```python
from build123d import *

# Parameters (mm, degrees)
F0_R         = 28.5
F0_R_2       = 18.5
F1_DEPTH     = 15
F2_R         = 28.5
F2_R_2       = 18.5
F3_DEPTH     = 5
F4_R         = 2
F4_R_2       = 11.2
F5_DEPTH     = 25
F7_DEPTH     = 65
F8_W         = 40
F8_H         = 5
F9_DEPTH     = 18
F10_R        = 3.2
F11_DEPTH    = 25
F12_W        = 18
F12_H        = 3
F13_DEPTH    = 60
F14_C1_SIZE2 = 60
F14_C1_SIZE  = 18
F14_C2_SIZE2 = 60
F14_C2_SIZE  = 18
F14_C3_SIZE2 = 60
F14_C3_SIZE  = 18
F14_C4_SIZE2 = 60
F14_C4_SIZE  = 18


# Not quite as in the source:
# - a pattern or mirror of a feature is missing from the dataset's text; its kind, count and spacing are read off the source's solid
# - a feature names something its author has since deleted; it is built from what else it names


with BuildPart() as f1:
    # F0 (on Top) → F1 (new body)
    with BuildSketch(Plane.XY):
        Circle(F0_R)
        Circle(F0_R_2, mode=Mode.SUBTRACT)
    extrude(amount=-F1_DEPTH)

    # F2 (on face) → F3 (join)
    with BuildSketch(Plane.XY):
        Circle(F2_R)
        Circle(F2_R_2, mode=Mode.SUBTRACT)
        Circle(F2_R_2)
    extrude(amount=F3_DEPTH)

    # F4 (on face) → F5 (cut)
    with BuildSketch(Plane.XY.offset(5)):
        with Locations((0, 14)):
            Circle(F4_R)
        Circle(F4_R_2)
        with Locations((-14, 0)):
            Circle(F4_R)
        with Locations((0, -14)):
            Circle(F4_R)
        with Locations((14, 0)):
            Circle(F4_R)
    extrude(amount=-F5_DEPTH, mode=Mode.SUBTRACT)

    # F6 (on face) → F7 (join)
    with BuildSketch(Plane(origin=(0, 0, -15), x_dir=(1, 0, 0), z_dir=(0, 0, -1))):
        with BuildLine():
            ThreePointArc((-20.3039405042, -20), (-28.5, 0), (-20.3039405042, 20))
            Line((-20.3039405042, 20), (-35.3039405042, 20))
            Line((-35.3039405042, 20), (-35.3039405042, -20))
            Line((-35.3039405042, -20), (-20.3039405042, -20))
        make_face()
        with BuildLine():
            Line((35.3039405042, 20), (20.3039405042, 20))
            ThreePointArc((20.3039405042, 20), (26.3715026532, 10.8071202369), (28.5, 0))
            ThreePointArc((28.5, 0), (26.3715026532, -10.8071202369), (20.3039405042, -20))
            Line((20.3039405042, -20), (35.3039405042, -20))
            Line((35.3039405042, -20), (35.3039405042, 20))
        make_face()
    extrude(amount=-F7_DEPTH)

    # F8 (on face) → F9 (join)
    with BuildSketch(Plane.YZ.offset(35.3039405042)):
        with Locations((0, 47.5)):
            Rectangle(F8_W, F8_H)
    f9 = extrude(amount=F9_DEPTH)

    # F9_copies: F9 across plane
    add(f9.mirror(Plane(origin=(0, 0, 0), x_dir=(0, 0, -1), z_dir=(-1, 0, 0))))

    # F10 (on face) → F11 (cut)
    with BuildSketch(Plane(origin=(0, 0, 45), x_dir=(1, 0, 0), z_dir=(0, 0, -1))):
        with Locations((44.9877695576, 12)):
            Circle(F10_R)
        with Locations((44.9877695576, -12)):
            Circle(F10_R)
    f11 = extrude(amount=-F11_DEPTH, mode=Mode.SUBTRACT)

    # F11_copies: F11 across plane
    add(f11.mirror(Plane(origin=(0, 0, 0), x_dir=(0, 0, -1), z_dir=(-1, 0, 0))), mode=Mode.SUBTRACT)

    # F12 (on face) → F13 (join)
    with BuildSketch(Plane(origin=(0, 0, 45), x_dir=(1, 0, 0), z_dir=(0, 0, -1))):
        with Locations((44.3039405042, 18.5)):
            Rectangle(F12_W, F12_H)
        with Locations((44.3039405042, -18.5)):
            Rectangle(F12_W, F12_H)
    f13 = extrude(amount=F13_DEPTH)

    # F13_copies: F13 across plane
    add(f13.mirror(Plane(origin=(0, 0, 0), x_dir=(0, 0, -1), z_dir=(-1, 0, 0))))

    # F14: chamfer of 60 x 18 on 4 edges, made by hand

    # F14_c1
    f14_c1_edges = [f1.edges().sort_by_distance(p)[0] for p in [
        (-53.3039405042, 18.5, -15),
    ]]
    f14_c1_side = f1.faces().sort_by_distance((-52.9439405042, 18.5, -15))[0]
    chamfer(f14_c1_edges, length=F14_C1_SIZE, length2=F14_C1_SIZE2, reference=f14_c1_side)

    # F14_c2
    f14_c2_edges = [f1.edges().sort_by_distance(p)[0] for p in [
        (-53.3039405042, -18.5, -15),
    ]]
    f14_c2_side = f1.faces().sort_by_distance((-52.9439405042, -18.5, -15))[0]
    chamfer(f14_c2_edges, length=F14_C2_SIZE, length2=F14_C2_SIZE2, reference=f14_c2_side)

    # F14_c3
    f14_c3_edges = [f1.edges().sort_by_distance(p)[0] for p in [
        (53.3039405042, -18.5, -15),
    ]]
    f14_c3_side = f1.faces().sort_by_distance((52.9439405042, -18.5, -15))[0]
    chamfer(f14_c3_edges, length=F14_C3_SIZE, length2=F14_C3_SIZE2, reference=f14_c3_side)

    # F14_c4
    f14_c4_edges = [f1.edges().sort_by_distance(p)[0] for p in [
        (53.3039405042, 18.5, -15),
    ]]
    f14_c4_side = f1.faces().sort_by_distance((52.9439405042, 18.5, -15))[0]
    chamfer(f14_c4_edges, length=F14_C4_SIZE, length2=F14_C4_SIZE2, reference=f14_c4_side)


solid = f1.part
```
Here's how the part is built. I have some questions about the finished solid (model axes, mm). A direction names the side the tool comes from. Give positions to 0.01 mm unless a question says otherwise; leave off trailing zeros. Loops run counter-clockwise (first coordinate to the right, second up) from the corner with the lowest first, then second, coordinate; pieces in that order, holes last. Notation, with made-up numbers: M 30.25,30.25 L 55.25,30.25 A14 cw 55.25,45.25 Z; hole C 35,-17.5 d8. An arc over 180 degrees is marked long. Return JSON: item names as keys, results as strings.
Item 1: Please list where these lines run through material, in increasing order: line 1 (Y direction, x = 0, z = 4.05); line 2 (X direction, y = -12, z = 47); line 3 (Y direction, x = -37, z = -3.5).
A:
{"line 1": "y = -28.5 to -16, -12 to -11.2, 11.2 to 12, 16 to 28.5", "line 2": "x = -53.3 to -48.19, -41.79 to -25.85, 25.85 to 41.79, 48.19 to 53.3", "line 3": "y = -20 to -17, 17 to 20"}
Item 2: Thinking about a two-plate mould opening in X: for faces 1 (the flat face through (35.304, 0, 15)), 2 (the cylindrical face through (-4.01, -18.06, -7.4)), 3 (the flat face through (-53.304, 0, 48)), 4 (the cylindrical face through (-47.94, 13.23, 47.46)), which applies, released by +X, released by -X, zero draft, split by the parting line, or undercut?
A:
{"face 1": "released by +X", "face 2": "undercut", "face 3": "released by -X", "face 4": "undercut"}
Item 3: Imagine slicing it at C-C on y = -14. List the corners of the cut face in (x, z) for me, then the cut area to 3 significant figures.
A:
{"outline": "M -53.3,45 L -47.49,45 L -47.49,50 L -53.3,50 Z; M -42.49,45 L -35.3,45 L -35.3,-15 L -12.09,-15 L -12.09,0 L -2,0 L -2,5 L -24.82,5 L -24.82,50 L -42.49,50 Z; M 2,0 L 12.09,0 L 12.09,-15 L 35.3,-15 L 35.3,45 L 42.49,45 L 42.49,50 L 24.82,50 L 24.82,5 L 2,5 Z; M 47.49,45 L 53.3,45 L 53.3,50 L 47.49,50 Z", "area": "2,100 mm^2"}
Item 4: Imagine slicing it at B-B on x = -14. List the corners of the cut face in (y, z) for me, then the cut area to 3 significant figures.
A:
{"outline": "M -24.82,-15 L -12.09,-15 L -12.09,0 L -2,0 L -2,5 L -24.82,5 Z; M 2,0 L 12.09,0 L 12.09,-15 L 24.82,-15 L 24.82,5 L 2,5 Z", "area": "610 mm^2"}
Item 5: On a 3-axis mill with a long thin cutter (end or side, diameter ignored), from which of +Z, -Z, +X, -X, +Y, -Y can I reach the whole of each face in a straight line? I mean faces 5 (the flat face through (-35.304, 0, 15)), 6 (the flat face through (44, 0, 45)), 7 (the flat face through (33, 20, 24)), 8 (the flat face through (8, 8.5, 0)). Say none if no direction works.
A:
{"face 5": "-Z, -X", "face 6": "-Z, +X", "face 7": "+Z, -Z, +X, +Y", "face 8": "-Z"}
Item 6: I'm going to push flat-ended pins straight in: pin 1 Ø5 at (x, y) = (0, -14) entering from -Z; pin 2 Ø12 at (y, z) = (22.5, 2.5) entering from +X; pin 3 Ø17 at (y, z) = (5.5, 13) entering from +X; pin 4 Ø6 at (x, y) = (44.99, 12) entering from +Z. Where does each tip first touch, or does it pass through?
A:
{"pin 1": "stops at z = 0", "pin 2": "stops at x = 42.19", "pin 3": "stops at x = 35.3", "pin 4": "passes through"}
Item 7: Imagine slicing it at D-D on y = 4. List the corners of the cut face in (x, z) for me.
A:
{"outline": "M -53.3,45 L -35.3,45 L -35.3,-15 L -18.06,-15 L -18.06,0 L -10.46,0 L -10.46,5 L -28.22,5 L -28.22,50 L -53.3,50 Z; M 10.46,0 L 18.06,0 L 18.06,-15 L 35.3,-15 L 35.3,45 L 53.3,45 L 53.3,50 L 28.22,50 L 28.22,5 L 10.46,5 Z"}
Item 8: Imagine slicing it at A-A on x = 0. List the corners of the cut face in (y, z) for me.
A:
{"outline": "M -28.5,-15 L -18.5,-15 L -18.5,0 L -16,0 L -16,5 L -28.5,5 Z; M -12,0 L -11.2,0 L -11.2,5 L -12,5 Z; M 11.2,0 L 12,0 L 12,5 L 11.2,5 Z; M 16,0 L 18.5,0 L 18.5,-15 L 28.5,-15 L 28.5,5 L 16,5 Z"}
